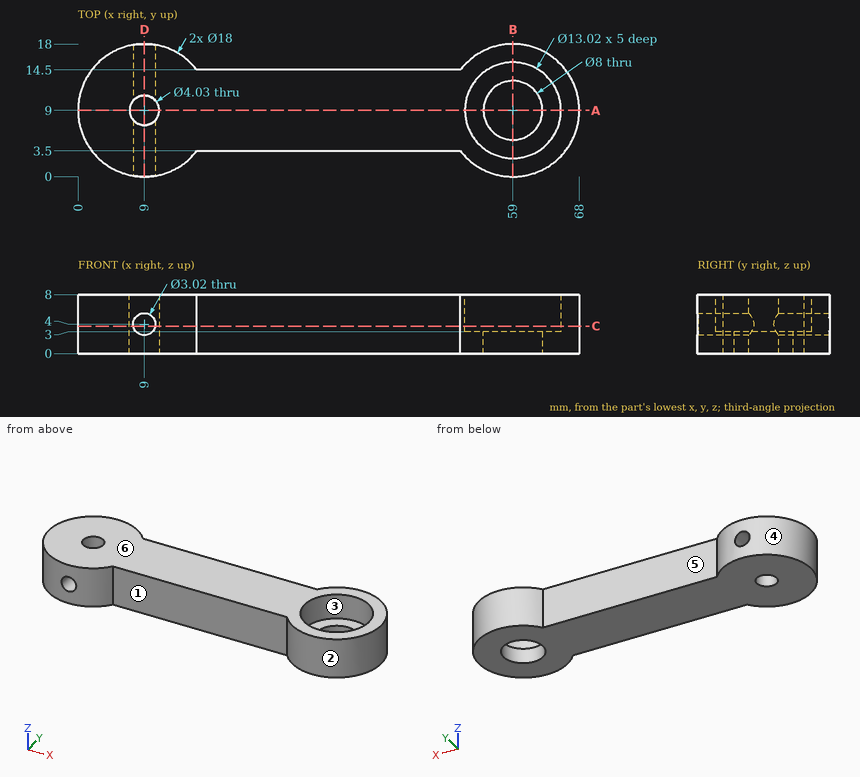
Job drawing, mm, ordinate dimensions from the low corner. One solid piece. A direction names the side the tool comes from. Round coordinates to 2 decimals unless told otherwise and drop trailing zeros. Loops run counter-clockwise (first coordinate to the right, second up) from the corner with the lowest first, then second, coordinate; pieces in that order, holes last. Notation, with made-up numbers: (34, -20.75) -> (59, -20.75) arc R25 ccw to (59, -0.75) -> close; hole circle Ø1 at (56.5, -3.5). An arc over 180 degrees is marked (long way). One line per item, written item: value. Start each with the question number.
Q1. Probe line 1 along Y through (x, z) = (59, 5.75); line 2 along X through (y, z) = (6, 4); line 3 along X through (y, z) = (7.75, 6.75). List the from-to ranges inside material, lowest first.
Q2. Drop flat-ended pins along their axis: pin 1 Ø1 at (y, z) = (3.5, 1) entering from -X; pin 2 Ø2.5 at (x, z) = (28.5, 4.5) entering from +Y; pin 3 Ø3 at (x, y) = (9, 9) entering from -Z; pin 4 Ø1 at (y, z) = (4, 3.5) entering from -X. Give the stop position or say it passes through.
Q3. Cut at D-D on x = 9. List the corners of the cut face in (y, z) (3 decimals), plus the area to 3 significant figures.
Q4. Cut at A-A on y = 9. List the corners of the cut face in (x, z) (3 decimals).
Q5. 3-axis set-ups, long thin cutter, end or side, ignore diameter. For the marked faces 1, 2 and 3: which of +Z, -Z, +X, -X, +Y, -Y reach the whole face in a straight line?
Q6. Two-plate mould, pull along X, no slides. Class the marked faces 4, 5 and 6: released by +X, released by -X, zero draft, split by the parting line, or undercut.
Q7. Cut at C-C on z = 3.75. List the corners of the cut face in (x, y) (3 decimals).
Q8. Cut at B-B on x = 59. List the corners of the cut face in (y, z), plus the area to 3 significant figures.
Computed:
1. line 1: 0 to 2.49, 15.51 to 18
1. line 2: 0.51 to 7.49, 10.51 to 53.22, 64.78 to 67.49
1. line 3: 0.09 to 7.42, 10.58 to 52.61, 65.39 to 67.91
2. pin 1: x = 1.52
2. pin 2: y = 14.5
2. pin 3: through
2. pin 4: x = 1.21
3. outline: (0, 0) -> (6.985, 0) -> (6.985, 2.49) -> (0, 2.49) -> close; (0, 5.51) -> (6.985, 5.51) -> (6.985, 8) -> (0, 8) -> close; (11.015, 0) -> (18, 0) -> (18, 2.49) -> (11.015, 2.49) -> close; (11.015, 5.51) -> (18, 5.51) -> (18, 8) -> (11.015, 8) -> close
3. area: 69.6 mm²
4. outline: (0, 0) -> (6.985, 0) -> (6.985, 8) -> (0, 8) -> close; (11.015, 0) -> (55, 0) -> (55, 3) -> (52.49, 3) -> (52.49, 8) -> (11.015, 8) -> close; (63, 0) -> (68, 0) -> (68, 8) -> (65.51, 8) -> (65.51, 3) -> (63, 3) -> close
5. face 1: +Z, -Z, -Y
5. face 2: +Z, -Z
5. face 3: +Z
6. face 4: undercut
6. face 5: undercut
6. face 6: zero draft
7. outline: (7.511, 0.124) -> (7.511, 7.643) arc R2.015 cw to (7.511, 10.357) -> (7.511, 17.876) arc R9 ccw to start; (10.489, 0.124) arc R9 ccw to (16.124, 3.5) -> (51.876, 3.5) arc R9 ccw (long way) to (51.876, 14.5) -> (16.124, 14.5) arc R9 ccw to (10.489, 17.876) -> (10.489, 10.357) arc R2.015 cw to (10.489, 7.643) -> close; hole circle Ø13.02 at (59, 9)
8. outline: (0, 0) -> (5, 0) -> (5, 3) -> (2.49, 3) -> (2.49, 8) -> (0, 8) -> close; (13, 0) -> (18, 0) -> (18, 8) -> (15.51, 8) -> (15.51, 3) -> (13, 3) -> close
8. area: 54.9 mm²
